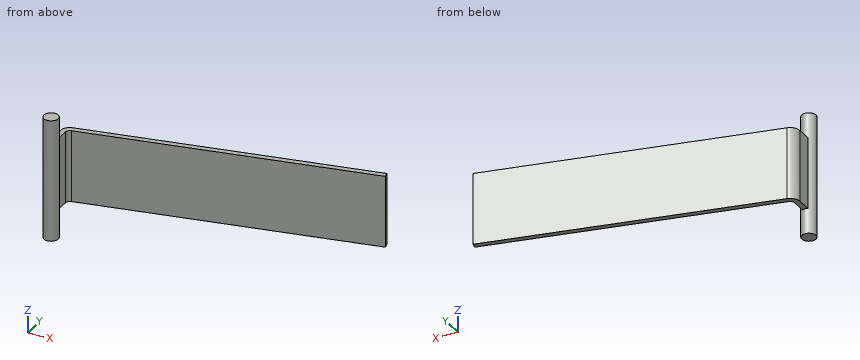
from build123d import *

# Parameters (mm, degrees)
SKETCH2_W           = 0.3
SKETCH2_H           = 4
SKETCH4_R           = 0.4
BOSS_EXTRUDE1_DEPTH = 3.4


with BuildPart() as part:
    # Sweep1: sweep along a path in Sketch1
    with BuildLine(Plane.XY) as sweep1_path:
        Line((0, 0), (0, 1.178041516))
        ThreePointArc((0, 1.178041516), (0.08839809, 1.428848712), (0.314521248, 1.568801523))
        Line((0.314521248, 1.568801523), (16, 5))
    # Sketch2 → Sweep1 (sweep)
    with BuildSketch(Plane(origin=(0, 0, 0), x_dir=(1, 0, 0), z_dir=(0, 1, 0))):
        Rectangle(SKETCH2_W, SKETCH2_H)
    sweep(path=sweep1_path.line)

    # Sketch4 → Boss-Extrude1 (add, symmetric)
    with BuildSketch(Plane.XY):
        Circle(SKETCH4_R)
    extrude(amount=BOSS_EXTRUDE1_DEPTH, both=True)


solid = part.part
Geometry: final body of the model. Coordinates: model frame, mm. Round coordinates to 2 decimals unless told otherwise and drop trailing zeros. Loops run counter-clockwise (first coordinate to the right, second up) from the corner with the lowest first, then second, coordinate; pieces in that order, holes last. Notation, with made-up numbers: M 75,56.25 L 128,56.25 A27 cw 128,94.25 Z; hole C 55.5,-8 d1. An arc over 180 degrees is marked long. Put each result on its own line as item: value. Start each with the question number.
(1) Section query C-C (y = 0). Return loops of the section in (x, z).
(2) Contact query for flat-ended pins moving along their axis: pin 1 Ø1.5 at (y, z) = (0.5, -1) entering from +X; pin 2 Ø1.4 at (x, y) = (5.5, 2.5) entering from -Z; pin 3 Ø0.6 at (y, z) = (1, 0) entering from -X; pin 4 Ø2.5 at (x, y) = (10.5, 2) entering from +Z. Output: stop coordinate, or through.
(3) Section query B-B (x = 0). Return loops of the section in (y, z), then the cut area to 3 significant figures.
(4) Material intervals for line 1 along Z through (x, y) = (14.75, 4.7); line 2 along X through (y, z) = (1.05, 1.25); line 3 along Y through (x, z) = (3.25, 0.75), sorted ascending. Write a range as [from, to].
(5) Section query A-A (z = 0.75). Return loops of the section in (x, y), then the cut area to 3 significant figures.
(6) Section query D-D (y = 1). Return loops of the section in (x, z).
Findings below:
1. outline: M -0.4,-3.4 L 0.4,-3.4 L 0.4,3.4 L -0.4,3.4 Z
2. pin 1: stops at x = 0.4
2. pin 2: stops at z = -2
2. pin 3: stops at x = -0.15
2. pin 4: passes through
3. outline: M -0.4,-3.4 L 0.4,-3.4 L 0.4,-2 L 1.56,-2 L 1.56,2 L 0.4,2 L 0.4,3.4 L -0.4,3.4 Z
3. area: 10.1 mm2
4. line 1: z = [-2, 2]
4. line 2: x = [-0.15, 0.15]
4. line 3: y = [2.06, 2.36]
5. outline: M -0.15,0.37 A0.4 ccw long 0.15,0.37 L 0.15,1.18 A0.25 cw 0.35,1.42 L 16.03,4.85 L 15.97,5.15 L 0.28,1.72 A0.55 ccw -0.15,1.18 Z
5. area: 5.72 mm2
6. outline: M -0.15,-2 L 0.15,-2 L 0.15,2 L -0.15,2 Z
